```python
from build123d import *

# Parameters (mm, degrees)
S01_TENDON_CAPTIVE_TAIL_R                      = 0.6
F_01_TENDON_CAPTIVE_TAIL_DEPTH                 = 12
S02_CROSSED_TENDON_R                           = 0.6
F_02_CROSSED_TENDON_DEPTH                      = 33.010681761
S03_TENDON_THROUGH_REAR_GROMMET_R              = 0.6
F_03_TENDON_THROUGH_REAR_GROMMET_DEPTH         = 12
F_04_START                                     = -0.55
F_04_TENDON_RETURN_DEPTH                       = 1.1
F_05_START                                     = -0.55
F_05_REMOVABLE_BACKED_EYE_AROUND_POLISHE_DEPTH = 1.1
S06_DRESSED_EYE_KNOT_ENVELOPE_R                = 2
F_06_DRESSED_EYE_KNOT_ENVELOPE_DEPTH           = 8.5


with BuildPart() as part:
    # S01 - Tendon captive tail → 01 - Tendon captive tail (new body)
    with BuildSketch(Plane.XY.offset(25.959868809)):
        with Locations((5.619098901, -13.907757819)):
            Circle(S01_TENDON_CAPTIVE_TAIL_R)
    extrude(amount=F_01_TENDON_CAPTIVE_TAIL_DEPTH)

    # S02 - Crossed tendon → 02 - Crossed tendon (add)
    with BuildSketch(Plane(origin=(10.190970454, -0.54666496, -12.992860813), x_dir=(0.7871038979441459, 0.025929320968004606, 0.6162752016390648), z_dir=(-0.6168204388970357, 0.0330875378277926, 0.7864081389452698))):
        with Locations(Location((20.060619317, -14.986740778, 0), (0, 0, 266.097812634))):
            Circle(S02_CROSSED_TENDON_R)
    extrude(amount=F_02_CROSSED_TENDON_DEPTH)

    # S03 - Tendon through rear grommet → 03 - Tendon through rear grommet (add)
    with BuildSketch(Plane.XY.offset(-12)):
        with Locations(Location((25.980762114, -15, 0), (0, 0, 266.929477468))):
            Circle(S03_TENDON_THROUGH_REAR_GROMMET_R)
    extrude(amount=F_03_TENDON_THROUGH_REAR_GROMMET_DEPTH)

    # S04 - Tendon return → 04 - Tendon return (add)
    with BuildSketch(Plane(origin=(12.990381057, -22.5, 0), x_dir=(-0.8660254037844386, -0.5000000000000003, 0), z_dir=(0.5000000000000003, -0.8660254037844386, 0)).offset(F_04_START)):
        with BuildLine():
            Line((-14.4, 12), (-14.4, 45))
            ThreePointArc((-14.4, 45), (-17.211774901, 51.788225099), (-24, 54.6))
            Line((-24, 54.6), (-67.598500564, 54.6))
            Line((-67.598500564, 54.6), (-67.598500564, 53.4))
            Line((-67.598500564, 53.4), (-24, 53.4))
            ThreePointArc((-24, 53.4), (-18.060303038, 50.939696962), (-15.6, 45))
            Line((-15.6, 45), (-15.6, 12))
            Line((-15.6, 12), (-14.4, 12))
        make_face()
    extrude(amount=F_04_TENDON_RETURN_DEPTH)

    # S05 - Removable backed eye around polished clevis sleeve → 05 - Removable backed eye around polished clevis sleeve (add)
    with BuildSketch(Plane.XY.offset(-54).offset(F_05_START)):
        with BuildLine():
            Line((71.084194722, 11.675564254), (71.257399803, 11.775564254))
            ThreePointArc((71.257399803, 11.775564254), (76.926405229, 10.256558829), (75.407399803, 4.587553403))
            Line((75.407399803, 4.587553403), (65.881120362, -0.912446597))
            Line((65.881120362, -0.912446597), (59.259967939, -1.444274196))
            Line((59.259967939, -1.444274196), (53.745866324, 0.106429959))
            Line((53.745866324, 0.106429959), (54.211891727, 1.299250282))
            Line((54.211891727, 1.299250282), (59.552788262, -0.351453873))
            Line((59.552788262, -0.351453873), (65.807434334, 0.315181347))
            Line((65.807434334, 0.315181347), (74.857399803, 5.540181347))
            ThreePointArc((74.857399803, 5.540181347), (75.973777285, 9.706558829), (71.807399803, 10.82293631))
            Line((71.807399803, 10.82293631), (71.634194722, 10.72293631))
            Line((71.634194722, 10.72293631), (71.084194722, 11.675564254))
        make_face()
    extrude(amount=F_05_REMOVABLE_BACKED_EYE_AROUND_POLISHE_DEPTH)

    # S06 - Dressed eye knot envelope → 06 - Dressed eye knot envelope (add)
    with BuildSketch(Plane(origin=(38.623434459, 22.299250282, 0), x_dir=(0, 0, -1), z_dir=(0.8660254037844386, 0.5000000000000003, 0))):
        with Locations(Location((54, -25.980762114, 0), (0, 0, 90))):
            Circle(S06_DRESSED_EYE_KNOT_ENVELOPE_R)
    extrude(amount=F_06_DRESSED_EYE_KNOT_ENVELOPE_DEPTH)


solid = part.part
```
Can you work these out from the model? Positions are in its coordinate system, mm. A direction names the side the tool comes from. Round coordinates to 2 decimals unless told otherwise and drop trailing zeros. Order: outer loops, then holes, each group sorted by start corner. A loop starts at its lowest first (then second) coordinate and runs counter-clockwise, first axis right, second up. Notation, with made-up numbers: (84.25, 83) -> (142.25, 83) arc R26 ccw to (142.25, 103) -> close; hole circle Ø9 at (57, 56). An arc over 180 degrees is marked (long way). Return JSON: item names as keys, results as strings. Group by question number.
1. If we section it at D-D, the plane x = 45: Write out the boundary of the cut face in (y, z).
2. If we section it at A-A, the plane y = 9.5: Write out the boundary of the cut face in (x, z).
3. Which directions (+Z, -Z, +X, -X, +Y, -Y) give clear straight access to the entire face, cutting with the end or side of a thin tool? Please do faces 5 (the face through (58.989, 4.025, -54.861)), 6 (the face through (70.27, 2.89, -54.01)), 7 (the face through (70.711, 1.876, -54.008)).
4. If we section it at B-B, the plane x = 70: Write out the boundary of the cut face in (y, z), then the cut area to 3 significant figures.
5. I need wall thicknesses on line 1 (Z direction, x = 60.5, y = -1). Which ranges of the line are inside material? Lowest first, please. Write a range as [from, to].
6. Will these pins go through, and if not, where does the flat tip stop? pin 1 (5.5 mm diameter, centred on x = 43, y = -4.5, fed in from +Z); pin 2 (3.5 mm diameter, centred on x = 44.5, y = -6, fed in from -Z); pin 3 (12 mm diameter, centred on x = 27, z = 8.5, fed in from -Y).
7. If we section it at C-C, the plane z = -14.5: Write out the boundary of the cut face in (x, y), then the cut area to 3 significant figures.
8. We'd pull the mould along Y, two halves only. Please class faces 1 (the face through (27.8, -13.9, -51.7)), 2 (the face through (76.007, 9.648, -54.008)), 3 (the face through (65.2, 7.6, -54.6)), 4 (the face through (28.68, -13.43, -51)): released by +Y, released by -Y, zero draft, split by the parting line, or undercut.
Output values:
{
 "1": {"outline": "(-4.65, -54.6) -> (-3.38, -54.6) -> (-3.38, -53.4) -> (-4.65, -53.4) -> close"},
 "2": {"outline": "(67.32, -54.6) -> (69.52, -54.6) -> (69.52, -53.4) -> (67.32, -53.4) -> close; (76.08, -54.55) -> (77.27, -54.55) -> (77.27, -53.45) -> (76.08, -53.45) -> close"},
 "3": {"face 5": "none", "face 6": "+Z, -Z", "face 7": "+Z, -Z, +X, -Y"},
 "4": {"outline": "(1.47, -54.55) -> (2.74, -54.55) -> (2.74, -53.45) -> (1.47, -53.45) -> close; (9.78, -54.6) -> (11.05, -54.6) -> (11.05, -53.4) -> (9.78, -53.4) -> close", "area": "2.92 mm²"},
 "5": {"line 1": "[-54.55, -53.45]"},
 "6": {"pin 1": "z = -53.4", "pin 2": "z = -54.6", "pin 3": "y = -15.42"},
 "7": {"outline": "(25.19, -14.82) -> (25.74, -15.78) -> (26.78, -15.18) -> (26.23, -14.22) -> close", "area": "1.32 mm²"},
 "8": {"face 1": "released by -Y", "face 2": "undercut", "face 3": "zero draft", "face 4": "released by +Y"}
}
